For this review, use the dimensioned drawing (mm, ordinates from the lowest corner) and the shaded views. Coordinates: 2 decimals unless noted, no trailing zeros. Write each loop counter-clockwise with the first axis right and the second up, starting at its lowest first coordinate (ties: lowest second). Pieces come first, ordered by that corner, then holes. Notation, with made-up numbers: (13.25, -21.5) -> (43.25, -21.5) arc R11 cw to (43.25, -17.5) -> close; hole circle Ø2 at (67, 81). An arc over 180 degrees is marked (long way). Return JSON: item names as keys, results as strings. Group by question number.
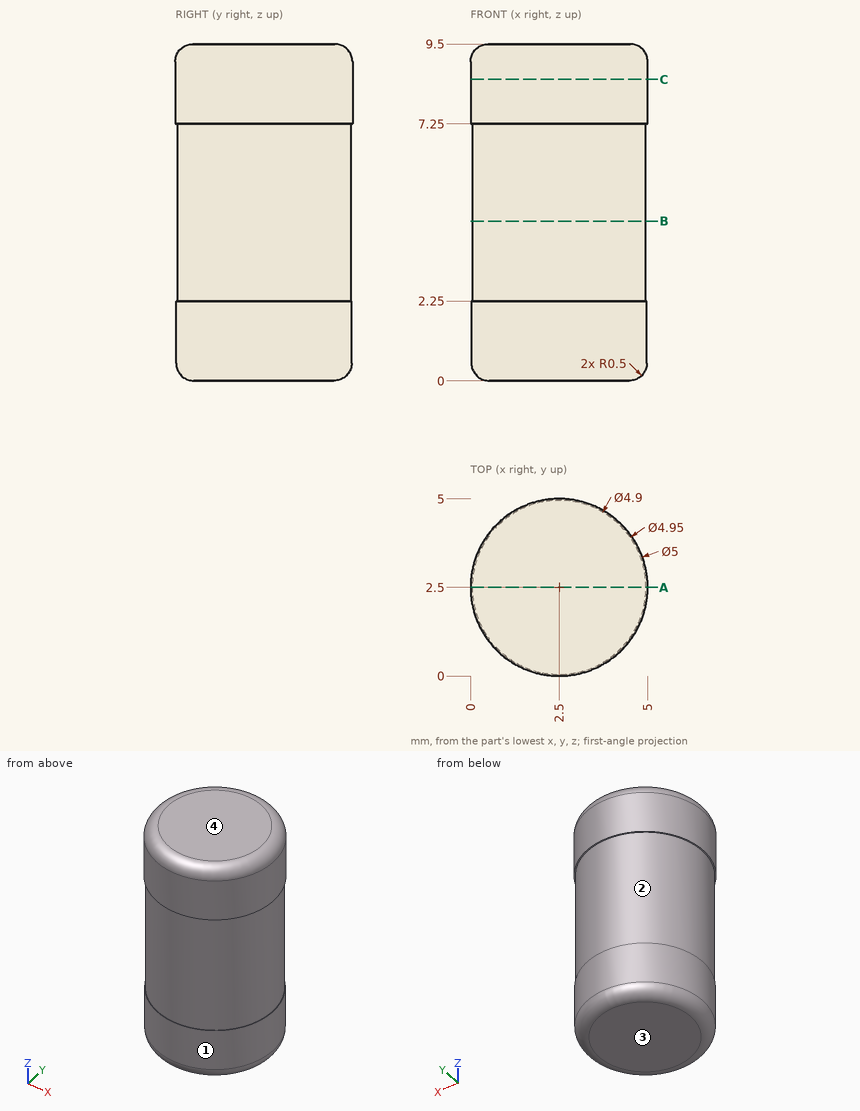
Q1. For P1, Ø1.5, axis at x = 4.5, z = 6, coming from the -Y side; P2, Ø3, axis at y = 4, z = 6.5, coming from the -X side; P3, Ø3, axis at y = 0.5, z = 2.5, coming from the -X side; P4, Ø2, axis at x = 1.5, z = 7, coming from the +Y side, all flat-tipped, find the tip position at first contact; note any pin that passes through.
Q2. Wall thickness on L1, parallel to X at y = 3, z = 7.75; L2, parallel to Y at x = 4.2, z = 1.75; L3, parallel to X at y = 0.3, z = 4.5: over which ranges is each line inside the solid? List them lowest first.
Q3. We need section B-B on z = 4.5. Write out the cut boundary in (x, y).
Q4. We need section C-C on z = 8.5. Write out the cut boundary in (x, y), plus the area to 3 significant figures.
Q5. We need section A-A on y = 2.5. Write out the cut boundary in (x, z) (3 decimals).
Q6. The part is to be moulded in two halves that separate along Z. For the marked faces 1, 2, 3 and 4, say which applies: +Z half, -Z half, draft (parallel to the pull), parting line (faces both ways), or undercut.
Findings below:
{
 "1": {"P1": "stops at y = 0.39", "P2": "stops at x = 0.01", "P3": "stops at x = 0.08", "P4": "stops at y = 5"},
 "2": {"L1": "x = 0.05 to 4.95", "L2": "y = 0.7 to 4.3", "L3": "x = 1.42 to 3.58"},
 "3": {"outline": "circle Ø4.9 at (2.5, 2.5)"},
 "4": {"outline": "circle Ø5 at (2.5, 2.5)", "area": "19.6 mm^2"},
 "5": {"outline": "(0, 7.25) -> (0.05, 7.25) -> (0.05, 2.25) -> (0.025, 2.25) -> (0.025, 0.5) arc R0.5 ccw to (0.525, 0) -> (4.475, 0) arc R0.5 ccw to (4.975, 0.5) -> (4.975, 2.25) -> (4.95, 2.25) -> (4.95, 7.25) -> (5, 7.25) -> (5, 9) arc R0.5 ccw to (4.5, 9.5) -> (0.5, 9.5) arc R0.5 ccw to (0, 9) -> close"},
 "6": {"face 1": "draft", "face 2": "undercut", "face 3": "-Z half", "face 4": "+Z half"}
}
